Source: CAD feature listing. Evaluate the final solid. Frame: model axes, mm. Face numbers are marked on the shaded views. A direction names the side the tool comes from. Give positions to 0.01 mm unless a question says otherwise; leave off trailing zeros. Loops run counter-clockwise (first coordinate to the right, second up) from the corner with the lowest first, then second, coordinate; pieces in that order, holes last. Notation, with made-up numbers: M 37,49 L 60,49 A25 ccw 60,67 Z; hole C 35.5,67 d9. An arc over 180 degrees is marked long. Put each result on its own line as item: value.
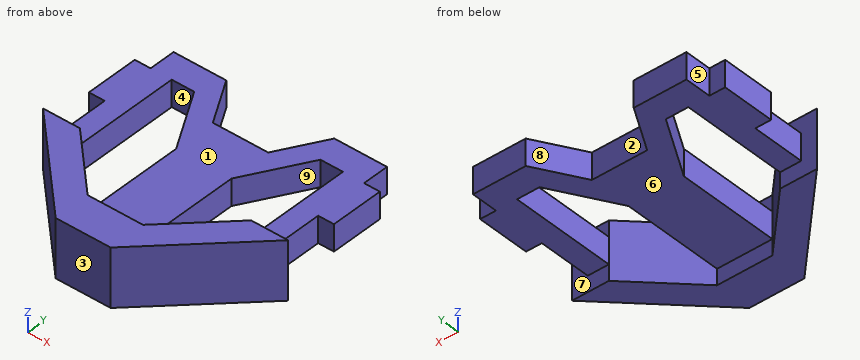
from build123d import *

# Parameters (mm, degrees)
EXTRUDE_1_DEPTH = 2.5
EXTRUDE_2_DEPTH = 5.5


with BuildPart() as part:
    # 草图1 → 凸台-拉伸1 (new, symmetric)
    with BuildSketch(Plane.XY):
        Polygon((-5.251410484, 27.285955328), (5.251410484, 27.285955328), (10.251410484, 35.946209366), (20.251410484, 35.946209366), (20.251410484, 30.946209366), (23.251410484, 30.946209366), (23.251410484, 20.946209366), (20.251410484, 20.946209366), (20.251410484, 10.946209366), (16.251410484, 10.946209366), (16.251410484, 30.946209366), (11.983461292, 30.946209366), (5.251410484, 19.285955328), (5.251410484, 0), (0, 0), (-5.251410484, 0), (-5.251410484, 19.285955328), (-11.983461292, 30.946209366), (-16.251410484, 30.946209366), (-16.251410484, 10.946209366), (-20.251410484, 10.946209366), (-20.251410484, 20.946209366), (-23.251410484, 20.946209366), (-23.251410484, 30.946209366), (-20.251410484, 30.946209366), (-20.251410484, 35.946209366), (-10.251410484, 35.946209366), align=None)
    extrude(amount=EXTRUDE_1_DEPTH, both=True)

    # 草图2 → 凸台-拉伸2 (add, symmetric)
    with BuildSketch(Plane.XY):
        Polygon((16.251410484, 10.946209366), (23.251410484, 10.946209366), (5.21701187, -7), (0, -7), (-5.21701187, -7), (-23.251410484, 10.946209366), (-16.251410484, 10.946209366), (-5.251410484, 0), (0, 0), (5.251410484, 0), align=None)
    extrude(amount=EXTRUDE_2_DEPTH, both=True)


solid = part.part
1. Section query B-B (y = 14). Output: boundary loops of the cut face in (x, z), plus the area to 3 significant figures.
Found:
outline: M -20.25,-2.5 L -16.25,-2.5 L -16.25,2.5 L -20.25,2.5 Z; M -5.25,-2.5 L 5.25,-2.5 L 5.25,2.5 L -5.25,2.5 Z; M 16.25,-2.5 L 20.25,-2.5 L 20.25,2.5 L 16.25,2.5 Z
area: 92.5 mm^2
2. Section query A-A (z = -0.5). State how many separate pieces and enclosed holes the cut face has, plus the area to 3 significant figures.
Found:
separate pieces: 1
enclosed holes: 2
area: 967 mm^2
3. Section query C-C (x = 11). Output: boundary loops of the cut face in (y, z), plus the area to 3 significant figures.
Found:
outline: M -1.25,-5.5 L 5.72,-5.5 L 5.72,5.5 L -1.25,5.5 Z; M 29.24,-2.5 L 35.95,-2.5 L 35.95,2.5 L 29.24,2.5 Z
area: 110 mm^2
4. Access query for the marked faces 5, 6, 7, 8 and 9. Directions: +Z, -Z, +X, -X, +Y, -Y. A direction counts if a zero-diameter tool reaches every point of the face in a straight line with its end or side. Return the directions, or none.
Found:
face 5: +Z, -Z, -X, +Y
face 6: -Z, +Y
face 7: +X
face 8: +Z, -Z, +Y
face 9: +Z, -Z
5. Draft query along Y for the marked faces 1, 2, 3 and 4. Return one class per face: pulls with the +Y half, pulls with the -Y half, needs draft (parallel to the pull), parting line crosses it, or undercut.
Found:
face 1: needs draft
face 2: pulls with the +Y half
face 3: pulls with the -Y half
face 4: undercut
6. Contact query for flat-ended pins moving along their axis: P1, Ø1.5, axis at x = 1, z = 0.5, coming from the +Y side; P2, Ø2.5, axis at x = 22.5, z = 0, coming from the -Y side; P3, Ø5, axis at x = -5, y = 9.5, coming from the -Z side. Output: stop coordinate, or through.
Found:
P1: y = 27.29
P2: y = 8.95
P3: z = -2.5
7. Section query D-D (z = 3.25). Output: boundary loops of the cut face in (x, y).
Found:
outline: M -23.25,10.95 L -5.22,-7 L 5.22,-7 L 23.25,10.95 L 16.25,10.95 L 5.25,0 L -5.25,0 L -16.25,10.95 Z
8. Material intervals for line 1 (X direction, y = 15, z = -2.25); line 2 (X direction, y = 10, z = 0.25); line 3 (Z direction, x = -17, y = 14), sorted ascending. Write a range as from..to.
Found:
line 1: -20.25..-16.25, -5.25..5.25, 16.25..20.25
line 2: -22.3..-15.3, -5.25..5.25, 15.3..22.3
line 3: -2.5..2.5
